For this review, use the dimensioned drawing (mm, ordinates from the lowest corner) and the shaded views. Round coordinates to 2 decimals unless told otherwise and drop trailing zeros. Order: outer loops, then holes, each group sorted by start corner. A loop starts at its lowest first (then second) coordinate and runs counter-clockwise, first axis right, second up. Notation, with made-up numbers: M 16,63 L 40,63 A22 cw 40,84 Z; hole C -9,86.25 d4. An arc over 180 degrees is marked long. Use a Markdown table: item, result. Add a question column.
1. To check wall thickness, follow probe 1 along X at (y, z) = (3.81, 0.8); probe 2 along Y at (x, z) = (2.5, 2.3) (1 decimal); probe 3 along Y at (x, z) = (40, 1.4) (1 decimal). State the ranges of each line that lie inside material, in increasing order.
2. Consider section D-D on x = 3. State the section outline as (y, z) points.
3. Consider section B-B on z = 1.2. Count the separate pieces of the cut face and the enclosed holes in it, then the cut area to 4 significant figures.
4. Consider section A-A on y = 21.59. State the section outline as (x, z) points.
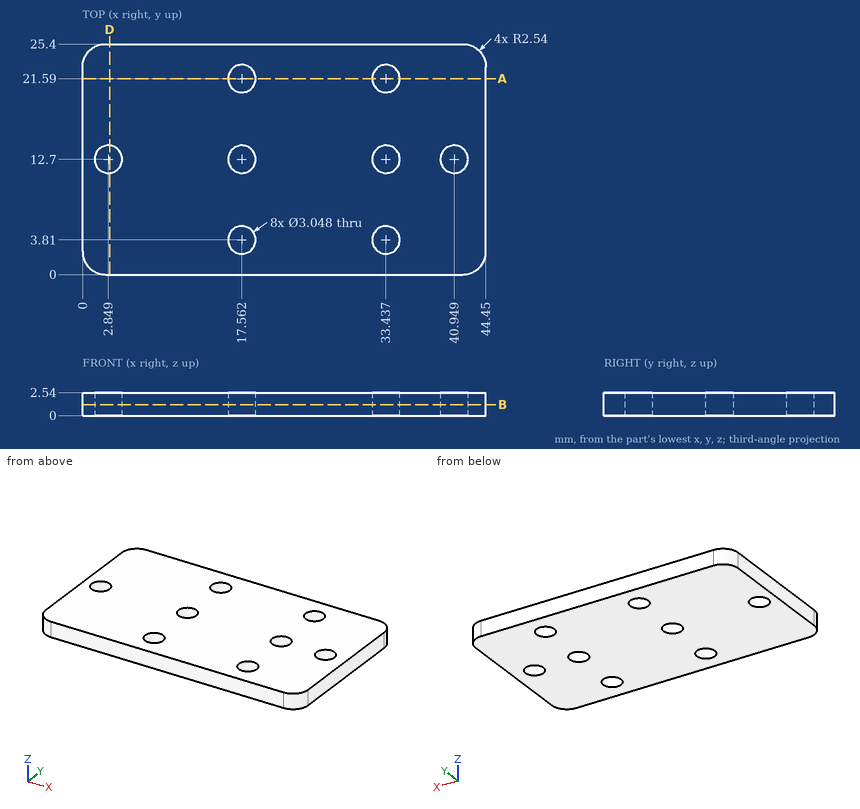
Answer block:
| question | item | result |
|---|---|---|
| 1 | probe 1 | 0 to 16.04, 19.09 to 31.91, 34.96 to 44.45 |
| 1 | probe 2 | 0 to 11.2, 14.2 to 25.4 |
| 1 | probe 3 | 0 to 11.5, 13.9 to 25.4 |
| 2 | outline | M 0,0 L 11.18,0 L 11.18,2.54 L 0,2.54 Z; M 14.22,0 L 25.4,0 L 25.4,2.54 L 14.22,2.54 Z |
| 3 | separate pieces | 1 |
| 3 | enclosed holes | 8 |
| 3 | area | 1,065 mm^2 |
| 4 | outline | M 0,0 L 16.04,0 L 16.04,2.54 L 0,2.54 Z; M 19.09,0 L 31.91,0 L 31.91,2.54 L 19.09,2.54 Z; M 34.96,0 L 44.45,0 L 44.45,2.54 L 34.96,2.54 Z |
